For this review, use the dimensioned drawing (mm, ordinates from the lowest corner) and the shaded views. A direction names the side the tool comes from. Coordinates: 2 decimals unless noted, no trailing zeros. Write each loop counter-clockwise with the first axis right and the second up, starting at its lowest first coordinate (ties: lowest second). Pieces come first, ordered by that corner, then holes.
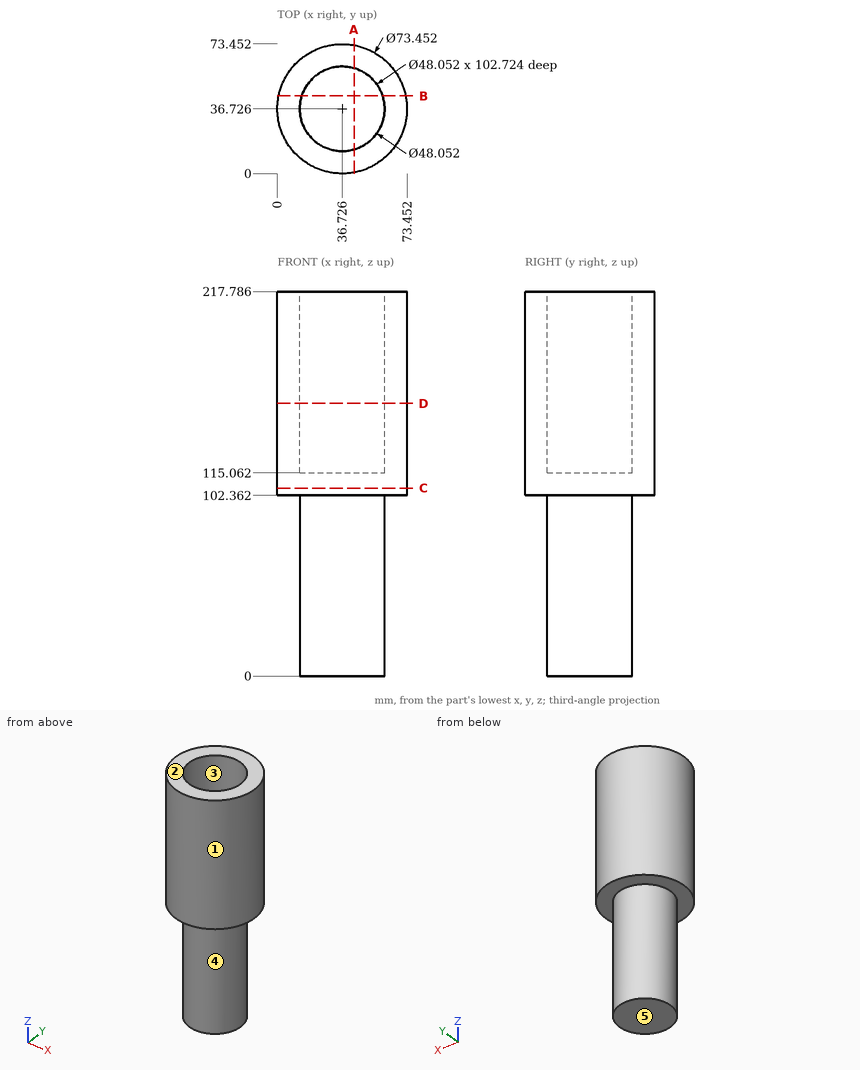
(1) Consider section C-C (z = 106.5). Give the boundary of the cut face in (x, y).
(2) Insertion check: pin 1 Ø6 at (x, z) = (38.5, 153.5) entering from -Y; pin 2 Ø14.5 at (x, y) = (47, 26) entering from +Z; pin 3 Ø1.5 at (x, z) = (16.5, 170) entering from -Y. Each pin has a flat end and moves straight along its axis. Give the tip position at first contact, or say it passes through.
(3) Wall thickness on line 1 (Z direction, x = 13, y = 17); line 2 (X direction, y = 38, z = 179); line 3 (Z direction, x = 35.5, y = 40): over which ranges is each line inside the solid? List them lowest first.
(4) Mouldability with a two-part tool opening along Y and no side actions: class the marked faces 1, 2 and 3 as +Y half, -Y half, draft (parallel to the pull), parting line (faces both ways), or undercut.
(5) Consider section D-D (z = 154.5). Give the boundary of the cut face in (x, y).
(6) Consider section B-B (y = 44). Give the boundary of the cut face in (x, z), plus the area to 3 significant figures.
(7) Consider section A-A (x = 43.5). Give the boundary of the cut face in (y, z) (1 decimal), plus the area to 3 significant figures.
(8) For the marked faces 4 and 5, list the 3-axis set-ups (+Z, -Z, +X, -X, +Y, -Y) from which the entire face can be reached by the end or side of a thin tool; tool diameter is ignored.
Results:
1. outline: circle Ø73.45 at (36.73, 36.73)
2. pin 1: stops at y = 0
2. pin 2: stops at z = 115.06
2. pin 3: stops at y = 5.59
3. line 1: z = 102.36 to 217.79
3. line 2: x = 0.02 to 12.73, 60.72 to 73.43
3. line 3: z = 0 to 115.06
4. face 1: parting line
4. face 2: draft
4. face 3: undercut
5. outline: circle Ø73.45 at (36.73, 36.73); hole circle Ø48.05 at (36.73, 36.73)
6. outline: (0.73, 102.36) - (13.83, 102.36) - (13.83, 0) - (59.62, 0) - (59.62, 102.36) - (72.72, 102.36) - (72.72, 217.79) - (59.62, 217.79) - (59.62, 115.06) - (13.83, 115.06) - (13.83, 217.79) - (0.73, 217.79) - close
6. area: 8,290 mm2
7. outline: (0.6, 102.4) - (13.7, 102.4) - (13.7, 0) - (59.8, 0) - (59.8, 102.4) - (72.8, 102.4) - (72.8, 217.8) - (59.8, 217.8) - (59.8, 115.1) - (13.7, 115.1) - (13.7, 217.8) - (0.6, 217.8) - close
7. area: 8,320 mm2
8. face 4: -Z
8. face 5: -Z, +X, -X, +Y, -Y
